from build123d import *

# Parameters (mm, degrees)
CROQUIS2_W              = 23
CROQUIS2_H              = 40
SALIENTE_EXTRUIR1_DEPTH = 50
CROQUIS3_W              = 17
CROQUIS3_H              = 34
CORTAR_EXTRUIR1_DEPTH   = 45
REDONDEO1_R             = 1
CROQUIS5_W              = 20
CROQUIS5_H              = 50
CROQUIS5_R              = 1.5
SALIENTE_EXTRUIR3_DEPTH = 3
REDONDEO2_R             = 1
CROQUIS8_W              = 10
CROQUIS8_H              = 48
SALIENTE_EXTRUIR4_DEPTH = 8
CROQUIS9_R              = 2.4
CORTAR_EXTRUIR2_DEPTH   = 75.067536749
REDONDEO3_R             = 1


with BuildPart() as part:
    # Croquis2 → Saliente-Extruir1 (new body)
    with BuildSketch(Plane(origin=(0, 0, 0), x_dir=(1, 0, 0), z_dir=(0, 1, 0))):
        with Locations((-11.5, 20)):
            Rectangle(CROQUIS2_W, CROQUIS2_H)
    extrude(amount=SALIENTE_EXTRUIR1_DEPTH)

    # Croquis3 → Cortar-Extruir1 (cut)
    with BuildSketch(Plane(origin=(0, 50, 0), x_dir=(1, 0, 0), z_dir=(0, 1, 0))):
        with Locations((-11.5, 20)):
            Rectangle(CROQUIS3_W, CROQUIS3_H)
    extrude(amount=-CORTAR_EXTRUIR1_DEPTH, mode=Mode.SUBTRACT)

    # Redondeo1
    redondeo1_edges = [part.edges().sort_by_distance(p)[0] for p in [
        (-11.5, 0, 0),
        (-23, 0, -20),
        (-11.5, 0, -40),
        (0, 0, -20),
        (0, 25, 0),
        (-23, 25, 0),
        (-23, 25, -40),
        (0, 25, -40),
    ]]
    fillet(redondeo1_edges, radius=REDONDEO1_R)

    # Croquis5 → Saliente-Extruir3 (add)
    # profile 1 of 2: a face of its own
    with BuildSketch(Plane(origin=(0, 0, 0), x_dir=(0, 0, -1), z_dir=(1, 0, 0))):
        with Locations((-1, 25)):
            Rectangle(CROQUIS5_W, CROQUIS5_H)
        with Locations((-6, 45)):
            Circle(CROQUIS5_R, mode=Mode.SUBTRACT)
        with Locations((-6, 5)):
            Circle(CROQUIS5_R, mode=Mode.SUBTRACT)
    # profile 2 of 2: a face of its own
    with BuildSketch(Plane(origin=(0, 0, 0), x_dir=(0, 0, -1), z_dir=(1, 0, 0))):
        with Locations((41, 25)):
            Rectangle(CROQUIS5_W, CROQUIS5_H)
        with Locations((46, 5)):
            Circle(CROQUIS5_R, mode=Mode.SUBTRACT)
        with Locations((46, 45)):
            Circle(CROQUIS5_R, mode=Mode.SUBTRACT)
    extrude(amount=-SALIENTE_EXTRUIR3_DEPTH)

    # Redondeo2
    redondeo2_edges = [part.edges().sort_by_distance(p)[0] for p in [
        (-12.5, 50, 0),
        (-22.707106781, 50, -0.292893219),
        (-23, 50, -20),
        (-22.707106781, 50, -39.707106781),
        (-12.5, 50, -40),
        (-3, 0, -45),
        (-3, 25, -51),
        (-3, 50, -45.5),
        (0, 25, -51),
        (0, 0, -41),
        (0, 0, 1),
        (0, 25, 11),
        (-3, 25, 11),
        (0, 50, -20),
        (-3, 50, 5.5),
        (-3, 0, 5),
    ]]
    fillet(redondeo2_edges, radius=REDONDEO2_R)

    # Croquis8 → Saliente-Extruir4 (add)
    with BuildSketch(Plane.ZY.offset(23)):
        with Locations((-29, 25)):
            Rectangle(CROQUIS8_W, CROQUIS8_H)
        with Locations((-11, 25)):
            Rectangle(CROQUIS8_W, CROQUIS8_H)
    extrude(amount=SALIENTE_EXTRUIR4_DEPTH)

    # Croquis9 → Cortar-Extruir2 (cut, through all)
    with BuildSketch(Plane.XY.offset(-6)):
        with Locations((-26.7, 28)):
            Circle(CROQUIS9_R)
        with Locations((-26.7, 36)):
            Circle(CROQUIS9_R)
        with Locations((-26.7, 44)):
            Circle(CROQUIS9_R)
    extrude(amount=-CORTAR_EXTRUIR2_DEPTH, mode=Mode.SUBTRACT)

    # Redondeo3
    redondeo3_edges = [part.edges().sort_by_distance(p)[0] for p in [
        (-31, 25, -34),
        (-31, 1, -29),
        (-31, 25, -24),
        (-31, 49, -29),
        (-31, 25, -6),
        (-31, 49, -11),
        (-31, 25, -16),
        (-31, 1, -11),
    ]]
    fillet(redondeo3_edges, radius=REDONDEO3_R)


solid = part.part
Can you work these out from the model? Positions are in its coordinate system, mm. A direction names the side the tool comes from. Give positions to 0.01 mm unless a question says otherwise; leave off trailing zeros. Order: outer loops, then holes, each group sorted by start corner. A loop starts at its lowest first (then second) coordinate and runs counter-clockwise, first axis right, second up. Notation, with made-up numbers: M -10,-35.5 L 6,-35.5 A9 cw 6,-28.5 Z; hole C -5.75,0 d7. An arc over 180 degrees is marked long. Use a Markdown table: item, result. Add a question column.
Item 1: We'd pull the mould along X, two halves only. Please class faces 1 (the flat face through (0, 25, -20)), 2 (the flat face through (-13, 25, 0)), 3 (the cylindrical face through (-27.22, 41.657, -28.93)): +X half, -X half, draft (parallel to the pull), parting line (faces both ways), or undercut.
Item 2: Suppose I cut it at D-D (z = -27). List the corners of the cut face in (x, y) for me, then the cut area to 3 significant figures.
Item 3: Suppose I cut it at A-A (x = -26.7). Count the separate pieces of the cut face and the enclosed holes in it, then the cut area to 3 significant figures.
Item 4: Will these pins go through, and if not, where does the flat tip stop? pin 1 (1.5 mm diameter, centred on x = -20, y = 9.5, fed in from -Z); pin 2 (2 mm diameter, centred on x = -27, y = 30.5, fed in from -Z); pin 3 (13.5 mm diameter, centred on x = -12.5, y = 16.5, fed in from +Z); pin 4 (5 mm diameter, centred on x = -10.5, z = -43.5, fed in from -Y).
Item 5: For faces 4 (the flat face through (-26, 1, -11)), 5 (the flat face through (-3, 28, -20)), 6 (the flat face through (-26, 25, -6)), which set-ups out of +Z, -Z, +X, -X, +Y, -Y let a thin tool reach every point of the face, with its end or its side?
Item 6: If I drill on L1, parallel to Z at x = -12, y = 31.5; L2, parallel to X at y = 22, z = -17.5; L3, parallel to Z at x = -24, y = 3.5, over which ranges is the centre line in solid material (lowest first)? Write a range as [from, to].
Item 7: Suppose I cut it at B-B (z = -46). List the corners of the cut face in (x, y) for me, then the cut area to 3 significant figures.
Answer sheet:
| question | item | result |
|---|---|---|
| 1 | face 1 | +X half |
| 1 | face 2 | draft |
| 1 | face 3 | undercut |
| 2 | outline | M -31,2 A1 ccw -30,1 L -23,1 A1 ccw -22,0 L -1,0 A1 ccw 0,1 L 0,49 A1 ccw -1,50 L -3,50 L -3,5 L -20,5 L -20,50 L -22,50 A1 ccw -23,49 L -30,49 A1 ccw -31,48 Z; hole C -26.7,28 d4.8; hole C -26.7,36 d4.8; hole C -26.7,44 d4.8 |
| 2 | area | 713 mm² |
| 3 | separate pieces | 8 |
| 3 | enclosed holes | 0 |
| 3 | area | 672 mm² |
| 4 | pin 1 | stops at z = -40 |
| 4 | pin 2 | stops at z = -34 |
| 4 | pin 3 | stops at z = 0 |
| 4 | pin 4 | passes through |
| 5 | face 4 | +Z, -Z, -X, -Y |
| 5 | face 5 | +Y |
| 5 | face 6 | +Z, -X, +Y, -Y |
| 6 | L1 | z = [-40, -37], [-3, 0] |
| 6 | L2 | x = [-23, -20], [-3, 0] |
| 6 | L3 | z = [-34, -24], [-16, -6] |
| 7 | outline | M -3,1 A1 ccw -2,0 L -1,0 A1 ccw 0,1 L 0,3.5 L -3,3.5 Z; M -3,6.5 L 0,6.5 L 0,43.5 L -3,43.5 Z; M -3,46.5 L 0,46.5 L 0,49 A1 ccw -1,50 L -2,50 A1 ccw -3,49 Z |
| 7 | area | 131 mm² |
